```python
from build123d import *

# Parameters (mm, degrees)
F1_DEPTH  = 247.65
F2_R      = 5.08
F3_R      = 38.1
F3_R_2    = 35.399063
F4_DEPTH  = 127
F5_R      = 127
F6_R      = 127
F7_R      = 63.5
F8_DEPTH  = 127
F9_W      = 381
F9_H      = 127
F10_DEPTH = 127
F11_R     = 50.8


with BuildPart() as f1:
    # F0 (on Front) → F1 (new body, symmetric)
    with BuildSketch(Plane.XZ):
        with BuildLine():
            Line((-1270, 0), (0, 0))
            Line((0, 0), (0, 48.26))
            Line((0, 48.26), (-1270, 48.26))
            ThreePointArc((-1270, 48.26), (-1317.048486, 64.613863), (-1343.809963, 106.623768))
            Line((-1343.809963, 106.623768), (-894.797157, 555.636574))
            Line((-894.797157, 555.636574), (-928.92213, 589.761548))
            Line((-928.92213, 589.761548), (-1377.934936, 140.748742))
            ThreePointArc((-1377.934936, 140.748742), (-1358.685059, 43.750751), (-1270, 0))
        make_face()
    extrude(amount=F1_DEPTH, both=True)

    # F2
    f2_edges = [f1.edges().sort_by_distance(p)[0] for p in [
        (-1377.934936, 0, 140.748742),
    ]]
    fillet(f2_edges, radius=F2_R)

    # F3 (on face) → F4 (cut)
    with BuildSketch(Plane(origin=(-759.341839, 0, 759.341839), x_dir=(0, -1, 0), z_dir=(-0.707107, 0, 0.707107))):
        with Locations((-95.25, -465.721811)):
            Circle(F3_R)
        with Locations((97.950937, -465.721811)):
            Circle(F3_R_2)
    extrude(amount=-F4_DEPTH, mode=Mode.SUBTRACT)

    # F5
    f5_edges = [f1.edges().sort_by_distance(p)[0] for p in [
        (0, -247.65, 24.13),
        (0, 247.65, 24.13),
    ]]
    fillet(f5_edges, radius=F5_R)

    # F6
    f6_edges = [f1.edges().sort_by_distance(p)[0] for p in [
        (-911.859644, -247.65, 572.699061),
        (-911.859644, 247.65, 572.699061),
    ]]
    fillet(f6_edges, radius=F6_R)

    # F7 (on face) → F8 (cut)
    with BuildSketch(Plane.XY.offset(48.26)):
        with Locations((-812.8, 0)):
            Circle(F7_R)
    extrude(amount=-F8_DEPTH, mode=Mode.SUBTRACT)

    # F9 (on face) → F10 (cut)
    with BuildSketch(Plane.XY.offset(48.26)):
        with Locations((-280.003726, 0)):
            Rectangle(F9_W, F9_H)
    extrude(amount=-F10_DEPTH, mode=Mode.SUBTRACT)

    # F11
    f11_edges = [f1.edges().sort_by_distance(p)[0] for p in [
        (-470.503726, 63.5, 24.13),
        (-470.503726, -63.5, 24.13),
        (-89.503726, 63.5, 24.13),
        (-89.503726, -63.5, 24.13),
    ]]
    fillet(f11_edges, radius=F11_R)


solid = f1.part
```
Could you check a few things on this model? Use its own coordinates, in mm. A direction names the side the tool comes from. Round coordinates to 2 decimals unless told otherwise and drop trailing zeros. Loops run counter-clockwise (first coordinate to the right, second up) from the corner with the lowest first, then second, coordinate; pieces in that order, holes last. Notation, with made-up numbers: (37, 2) -> (50, 2) arc R16 ccw to (50, 9) -> close; hole circle Ø4 at (21.25, 40). An arc over 180 degrees is marked (long way). Put each result on its own line as item: value.
Q1. I want a section at C-C on z = 416. Give the number of separate pieces and of enclosed holes in the cut face, and give its area (3 significant figures).
Checks:
separate pieces: 3
enclosed holes: 0
area: 24,600 mm2
Q2. I want a section at A-A on x = -812.8. Write out the boundary of the cut face in (y, z), and give its area (3 significant figures).
Checks:
outline: (-247.65, 0) -> (-63.5, 0) -> (-63.5, 48.26) -> (-247.65, 48.26) -> close; (63.5, 0) -> (247.65, 0) -> (247.65, 48.26) -> (63.5, 48.26) -> close
area: 17,800 mm2
Q3. I want a section at D-D on x = -1217. Write out the boundary of the cut face in (y, z), and give its area (3 significant figures).
Checks:
outline: (-247.65, 0) -> (247.65, 0) -> (247.65, 48.26) -> (-247.65, 48.26) -> close; (-247.65, 233.43) -> (247.65, 233.43) -> (247.65, 301.68) -> (-247.65, 301.68) -> close
area: 57,700 mm2
Q4. For pin 1 Ø12 at (x, y) = (-685.5, -104) entering from +Z; pin 2 Ø3 at (y, z) = (-131, 372.5) entering from +X; pin 3 Ø12.5 at (y, z) = (-1.5, 30.5) entering from -X, each with a flat end and sliding along its axis, tell me the tip position at first contact or that it passes through.
Checks:
pin 1: z = 48.26
pin 2: x = -1076.43
pin 3: x = -1352.85
Q5. Please list where these lines run through material, in increasing order: line 1 (Y direction, x = -812.8, z = 21); line 2 (Z direction, x = -1045, y = 145). Write a range as from..to.
Checks:
line 1: -247.65..-63.5, 63.5..247.65
line 2: 0..48.26, 405.43..473.68
Q6. I want a section at B-B on y = 0. Write out the boundary of the cut face in (x, z).
Checks:
outline: (-1378.29, 139.39) arc R111.76 ccw to (-1270, 0) -> (-876.3, 0) -> (-876.3, 48.26) -> (-1270, 48.26) arc R75.85 cw to (-1343.81, 106.62) -> (-894.8, 555.64) -> (-928.92, 589.76) -> (-1376.96, 141.72) arc R5.08 ccw to start; (-749.3, 0) -> (-470.5, 0) -> (-470.5, 48.26) -> (-749.3, 48.26) -> close; (-89.5, 0) -> (0, 0) -> (0, 48.26) -> (-89.5, 48.26) -> close
Q7. Thinking about a two-plate mould opening in X: for faces 1 (the flat face through (-1122.447, -3.467, 327.987)), 2 (the cylindrical face through (-1049.117, 74.768, 435.92)), 3 (the flat face through (-850, 247.65, 47)), which applies, pulls with the +X half, pulls with the -X half, needs draft (parallel to the pull), parting line crosses it, or undercut?
Checks:
face 1: pulls with the +X half
face 2: undercut
face 3: needs draft
Q8. Which directions (+Z, -Z, +X, -X, +Y, -Y) give clear straight access to the entire face, cutting with the end or side of a thin tool? Please do faces 4 (the cylindrical face through (-38.19, -211.435, 24.468)), 5 (the flat face through (-282, -63.5, 24)), 6 (the cylindrical face through (-1316.489, -3.467, 64.176)).
Checks:
face 4: +Z, -Z, +X, -Y
face 5: +Z, -Z
face 6: +X, +Y, -Y
